from build123d import *

# Parameters (mm, degrees)
SKETCH1_W                = 25
SKETCH1_H                = 6.75
BOSS_EXTRUDE1_DEPTH      = 6.5
BOSS_EXTRUDE4_DEPTH      = 6.5
BOSS_EXTRUDE3_DEPTH      = 6
BOSS_EXTRUDE3_DEPTH_BACK = 4.95
SKETCH4_W                = 2.3
SKETCH4_H                = 4.5
CUT_EXTRUDE1_DEPTH       = 23
SKETCH6_R                = 2.55
CUT_EXTRUDE2_DEPTH       = 10
BOSS_EXTRUDE5_DEPTH      = 1.575
CUT_EXTRUDE3_DEPTH       = 3
SKETCH9_R                = 0.8
CUT_EXTRUDE4_DEPTH       = 10.95
BOSS_EXTRUDE6_DEPTH      = 0.25


with BuildPart() as part:
    # Sketch1 → Boss-Extrude1 (new body)
    with BuildSketch(Plane(origin=(0, 0, 0), x_dir=(1, 0, 0), z_dir=(0, 1, 0))):
        with Locations((12.5, -3.375)):
            Rectangle(SKETCH1_W, SKETCH1_H)
    extrude(amount=BOSS_EXTRUDE1_DEPTH)

    # Sketch5 → Boss-Extrude4 (add)
    with BuildSketch(Plane(origin=(0, 6.5, 0), x_dir=(1, 0, 0), z_dir=(0, 1, 0))):
        Polygon((-5.715767665, -3.375), (-2.857883832, -8.325), (2.857883832, -8.325), (5.715767665, -3.375), (2.857883832, 1.575), (-2.857883832, 1.575), align=None)
    extrude(amount=-BOSS_EXTRUDE4_DEPTH)

    # Sketch3 → Boss-Extrude3 (add, two sides)
    with BuildSketch(Plane.XY.offset(3.375)) as boss_extrude3_sk:
        Polygon((21.275684175, 14.155521181), (26.183820092, 15.109566157), (30, -4.522977512), (25.091864083, -5.477022488), align=None)
    extrude(amount=BOSS_EXTRUDE3_DEPTH)
    extrude(boss_extrude3_sk.sketch, amount=-BOSS_EXTRUDE3_DEPTH_BACK)

    # Sketch4 → Cut-Extrude1 (cut)
    with BuildSketch(Plane(origin=(-1.876769127, 9.65514015, 0), x_dir=(0.981627183, 0.190808995, 0), z_dir=(-0.190808995, 0.981627183, 0))):
        with Locations((27.435790708, -2.675)):
            Rectangle(SKETCH4_W, SKETCH4_H)
    extrude(amount=-CUT_EXTRUDE1_DEPTH, mode=Mode.SUBTRACT)

    # Sketch6 → Cut-Extrude2 (cut)
    with BuildSketch(Plane(origin=(0, 6.5, 0), x_dir=(1, 0, 0), z_dir=(0, 1, 0))):
        with Locations((0, -3.335615973)):
            Circle(SKETCH6_R)
    extrude(amount=-CUT_EXTRUDE2_DEPTH, mode=Mode.SUBTRACT)

    # Sketch7 → Boss-Extrude5 (add)
    with BuildSketch(Plane(origin=(0, 0, -1.575), x_dir=(-1, 0, 0), z_dir=(0, 0, -1))):
        Polygon((-2.857883832, 0), (-24.027238758, 0), (-25.091864083, -5.477022488), (-30, -4.522977512), (-26.183820092, 15.109566157), (-21.275684175, 14.155521181), (-22.763766749, 6.5), (-2.857883832, 6.5), align=None)
    extrude(amount=-BOSS_EXTRUDE5_DEPTH)

    # Sketch8 → Cut-Extrude3 (cut)
    with BuildSketch(Plane(origin=(0, 0, 0), x_dir=(-1, 0, 0), z_dir=(0, -1, 0))):
        Polygon((-4.67653718, -11.475), (4.67653718, -11.475), (9.353074361, -3.375), (4.67653718, 4.725), (-4.67653718, 4.725), (-9.353074361, -3.375), align=None)
    extrude(amount=-CUT_EXTRUDE3_DEPTH, mode=Mode.SUBTRACT)

    # Sketch9 → Cut-Extrude4 (cut)
    with BuildSketch(Plane(origin=(0, 0, -1.575), x_dir=(-1, 0, 0), z_dir=(0, 0, -1))):
        with Locations((-28.437671168, -3.29858843)):
            Circle(SKETCH9_R)
        with Locations((-27.483626192, 1.609547487)):
            Circle(SKETCH9_R)
        with Locations((-26.529581215, 6.517683404)):
            Circle(SKETCH9_R)
        with Locations((-25.575536238, 11.425819321)):
            Circle(SKETCH9_R)
    extrude(amount=-CUT_EXTRUDE4_DEPTH, mode=Mode.SUBTRACT)

    # Sketch10 → Boss-Extrude6 (add)
    with BuildSketch(Plane.XY.offset(6.75)):
        Polygon((11.821517388, 5.121255448), (12.792571074, 5.121255448), (12.792571074, 1.621255448), (12.164365946, 1.621255448), (12.164365946, 4.537922115), (11.446417228, 4.537922115), align=None)
        Polygon((14.513825081, 5.121255448), (15.484878766, 5.121255448), (15.484878766, 1.621255448), (14.856673638, 1.621255448), (14.856673638, 4.537922115), (14.13872492, 4.537922115), align=None)
        Polygon((17.234878766, 5.210999038), (17.8182121, 5.210999038), (17.672378766, 4.537922115), (18.215748157, 5.013983814), (18.491289023, 4.537922115), (17.773340305, 4.335999038), (18.491289023, 4.134075961), (18.180692068, 3.647497435), (17.6541496, 4.134075961), (17.8182121, 3.460999038), (17.234878766, 3.460999038), (17.412262581, 4.134075961), (16.873801042, 3.647497435), (16.561801843, 4.134075961), (17.279750561, 4.335999038), (16.561801843, 4.537922115), (16.873801042, 5.036419711), (17.412262581, 4.537922115), align=None)
    extrude(amount=BOSS_EXTRUDE6_DEPTH)


solid = part.part
Read the model definition and answer for the solid it produces. Units are mm, in the model's axes. A direction names the side the tool comes from. Coordinates: 2 decimals unless noted, no trailing zeros. Order: outer loops, then holes, each group sorted by start corner. A loop starts at its lowest first (then second) coordinate and runs counter-clockwise, first axis right, second up. Notation, with made-up numbers: M 23.25,26.25 L 78.25,26.25 A18 ccw 78.25,59.25 Z; hole C -17.75,13.5 d3. An arc over 180 degrees is marked long. Put each result on its own line as item: value. Start each with the question number.
Item 1: Consider probe 1 along Z at (x, y) = (25.5, 7.75) (3 decimals); probe 2 along Z at (x, y) = (11, 2) (3 decimals); probe 3 along Z at (x, y) = (0, 3.5) (3 decimals). Determine where each line is inside the solid, lowest interval first. Write a range as [from, to].
Item 2: Section D-D, the plane z = 6.25 is taken. Determine the outline of the cut face in (x, y).
Item 3: Given pin 1 Ø1.4 at (x, y) = (28.44, -3.3) entering from -Z; pin 2 Ø1 at (y, z) = (12, 2) entering from +X; pin 3 Ø1.8 at (x, y) = (27, 1.5) entering from +Z (3 decimals); pin 4 Ø1 at (x, y) = (7, 4.5) entering from +Z, each flat-ended and moving along its own axis, determine where each tip first touches the part or whether it passes through.
Item 4: Section B-B, the plane z = 2.25 is taken. Determine the outline of the cut face in (x, y), plus the area to 3 significant figures.
Item 5: Section A-A, the plane x = 0 is taken. Determine the outline of the cut face in (y, z) (3 decimals), plus the area to 3 significant figures.
Item 6: Section C-C, the plane y = -0.75 is taken. Determine the outline of the cut face in (x, z) (3 decimals).
Item 7: The mould has two halves that part along X. Classify faces 1 (the face through (8, 6.5, 3)), 2 (the face through (-4.27, 4.77, 0.87)), 3 (the face through (17.5, 4.3, 7)), 4 (the face through (28.065, 5.431, -0.561)): +X half, -X half, draft (parallel to the pull), parting line (faces both ways), or undercut.
Item 8: For faces 5 (the face through (2.432, 4.774, 2.57)), 6 (the face through (15, 0, 3)), 7 (the face through (3.306, 4.774, 7.549)), 8 (the face through (27, 5, 4.925)), 9 (the face through (0, 5, 8.325)), determine the directions among +Z, -Z, +X, -X, +Y, -Y from which every point of the face is accessible in a straight line to the end or side of a thin tool.
Computed:
1. probe 1: z = [-1.575, 0.425], [4.925, 9.375]
1. probe 2: z = [-1.575, 6.75]
1. probe 3: z = [-1.575, 0.786], [5.886, 8.325]
2. outline: M -4.06,3 L 7.69,3 L 7.69,0 L 24.03,0 L 25.09,-5.48 L 30,-4.52 L 26.18,15.11 L 21.28,14.16 L 22.76,6.5 L -4.06,6.5 Z; hole C 25.58,11.43 d1.6; hole C 26.53,6.52 d1.6; hole C 27.48,1.61 d1.6; hole C 28.44,-3.3 d1.6
3. pin 1: passes through
3. pin 2: stops at x = 24.54
3. pin 3: stops at z = 9.375
3. pin 4: stops at z = 6.75
4. outline: M -5.07,3 L -2.31,3 L -2.31,6.5 L -5.07,6.5 Z; M 2.31,3 L 8.7,3 L 8.7,0 L 24.03,0 L 25.09,-5.48 L 27.74,-4.96 L 23.93,14.67 L 21.28,14.16 L 22.76,6.5 L 2.31,6.5 Z
4. area: 182 mm2
5. outline: M 3,-1.575 L 6.5,-1.575 L 6.5,0.786 L 3,0.786 Z; M 3,5.886 L 6.5,5.886 L 6.5,8.325 L 3,8.325 Z
5. area: 16.8 mm2
6. outline: M 24.173,-1.575 L 29.267,-1.575 L 29.267,0.425 L 26.924,0.425 L 26.924,4.925 L 29.267,4.925 L 29.267,9.375 L 24.173,9.375 Z
7. face 1: draft
7. face 2: -X half
7. face 3: undercut
7. face 4: +X half
8. face 5: +Y, -Y
8. face 6: +Z, -Z, -X, -Y
8. face 7: +Z, +Y, -Y
8. face 8: +X, +Y
8. face 9: +Z, -X, +Y, -Y
